from build123d import *

# Parameters (mm, degrees)
SKETCH1_W           = 14.5
SKETCH1_H           = 14.5
BOSS_EXTRUDE1_DEPTH = 24.6
CUT_EXTRUDE1_DEPTH  = 10
SKETCH4_R           = 4
BOSS_EXTRUDE2_DEPTH = 2
FILLET1_R           = 0.5
SKETCH6_W           = 8.45
SKETCH6_H           = 14.5
BOSS_EXTRUDE3_DEPTH = 5
SKETCH7_W           = 6
SKETCH7_H           = 2
CUT_EXTRUDE2_DEPTH  = 5
SKETCH8_R           = 0.55
CUT_EXTRUDE3_DEPTH  = 33.586807146
SKETCH9_R           = 1
CUT_EXTRUDE4_DEPTH  = 29.855891946


with BuildPart() as part:
    # Sketch1 → Boss-Extrude1 (new body)
    with BuildSketch(Plane(origin=(0, 0, 0), x_dir=(1, 0, 0), z_dir=(0, 1, 0))):
        Rectangle(SKETCH1_W, SKETCH1_H)
    extrude(amount=BOSS_EXTRUDE1_DEPTH)

    # Sketch2 → Cut-Extrude1 (cut, symmetric)
    with BuildSketch(Plane(origin=(0, 0, 0), x_dir=(0, 0, -1), z_dir=(1, 0, 0))):
        Polygon((-2, 24.6), (2, 24.6), (4.020725942, 21.1), (-4.020725942, 21.1), align=None)
    extrude(amount=CUT_EXTRUDE1_DEPTH, both=True, mode=Mode.SUBTRACT)

    # Sketch4 → Boss-Extrude2 (add)
    with BuildSketch(Plane.XZ):
        with Locations(Location((0, 0, 0), (0, 0, 270))):
            Circle(SKETCH4_R)
    extrude(amount=BOSS_EXTRUDE2_DEPTH)

    # Sketch3 → Cut-Revolve1 (revolve, cut)
    with BuildSketch(Plane(origin=(0, 0, 0), x_dir=(0, 0, -1), z_dir=(1, 0, 0))):
        with BuildLine():
            Line((3.302, 0), (3.302, -3.302))
            Line((3.302, -3.302), (0, -3.302))
            Line((0, -3.302), (0, 0))
            Line((0, 0), (0, 3.302))
            ThreePointArc((0, 3.302), (2.334866591, 2.334866591), (3.302, 0))
        make_face()
    revolve(axis=Axis((0, 0, 0), (0, 1, 0)), mode=Mode.SUBTRACT)

    # Fillet1
    fillet1_edges = [part.edges().sort_by_distance(p)[0] for p in [
        (0, 24.6, 2),
        (0, 24.6, -2),
        (0, 21.1, -4.020725942),
        (0, 21.1, 4.020725942),
    ]]
    fillet(fillet1_edges, radius=FILLET1_R)

    # Sketch6 → Boss-Extrude3 (add)
    with BuildSketch(Plane(origin=(0, 0, 0), x_dir=(1, 0, 0), z_dir=(0, 1, 0))):
        with Locations((11.475, 0)):
            Rectangle(SKETCH6_W, SKETCH6_H)
        with Locations((-11.475, 0)):
            Rectangle(SKETCH6_W, SKETCH6_H)
    extrude(amount=BOSS_EXTRUDE3_DEPTH)

    # Sketch7 → Cut-Extrude2 (cut)
    with BuildSketch(Plane.XZ):
        with Locations((10.7, 4.125)):
            Rectangle(SKETCH7_W, SKETCH7_H)
        with Locations((-10.7, -4.125)):
            Rectangle(SKETCH7_W, SKETCH7_H)
    extrude(amount=-CUT_EXTRUDE2_DEPTH, mode=Mode.SUBTRACT)

    # Sketch8 → Cut-Extrude3 (cut, through all)
    with BuildSketch(Plane(origin=(0, 0, -7.25), x_dir=(-1, 0, 0), z_dir=(0, 0, -1))):
        with Locations((-10.7, 2.5)):
            Circle(SKETCH8_R)
        with Locations((10.7, 2.5)):
            Circle(SKETCH8_R)
    extrude(amount=-CUT_EXTRUDE3_DEPTH, mode=Mode.SUBTRACT)

    # Sketch9 → Cut-Extrude4 (cut, through all)
    with BuildSketch(Plane(origin=(0, 21.1, 0), x_dir=(1, 0, 0), z_dir=(0, 1, 0))):
        with Locations(Location((0, 0, 0), (0, 0, 270))):
            Circle(SKETCH9_R)
    extrude(amount=-CUT_EXTRUDE4_DEPTH, mode=Mode.SUBTRACT)


solid = part.part
For this review, take the finished solid that the model builds, in its own axes (mm). A direction names the side the tool comes from. Give positions to 0.01 mm unless a question says otherwise; leave off trailing zeros. Loops run counter-clockwise (first coordinate to the right, second up) from the corner with the lowest first, then second, coordinate; pieces in that order, holes last. Notation, with made-up numbers: M 10.25,-1.5 L 63.25,-1.5 A22 cw 63.25,18.5 Z; hole C 86,36.25 d10. An arc over 180 degrees is marked long. Answer as a JSON object with one key per item and string values. Group by question number.
Q1. Tool access review of faces 5 (the flat face through (-7.7, 2, -4)), 6 (the flat face through (-7.25, 15, 0)), 7 (the flat face through (7.25, 15, 0)), 8 (the flat face through (0.101, 22.836, 3.018)), 9 (the cylindrical face through (-3.905, -0.986, 0.867)): name each direction out of +Z, -Z, +X, -X, +Y, -Y from which nothing blocks a thin tool from reaching the whole face with its end or side.
Q2. Add section A-A on z = 0. Give the boundary of the cut face in (x, y).
Q3. Add section B-B on x = 10.7. Give the boundary of the cut face in (y, z) (3 decimals), and give its area (4 significant figures).
Q4. Add section C-C on z = 4.5. Give the boundary of the cut face in (x, y).
Q5. Mouldability with a two-part tool opening along Y and no side actions: class faces 1 (the flat face through (-12, 5, 2)), 2 (the flat face through (0.101, 22.864, -3.002)), 3 (the flat face through (0.1, 21.1, 1.4)), 4 (the flat face through (0, 9, 7.25)) as +Y half, -Y half, draft (parallel to the pull), parting line (faces both ways), or undercut.
Q6. Insertion check: P1, Ø1.8, axis at x = -10.7, y = 2.5, coming from the +Z side; P2, Ø1, axis at x = 3.5, z = 3, coming from the -Y side; P3, Ø7, axis at y = 19, z = 3.5, coming from the -X side; P4, Ø2, axis at y = 19.5, z = -0.5, coming from the +X side. Each pin has a flat end and moves straight along its axis. Give the tip position at first contact, or say it passes through.
Q7. Add section D-D on x = -12. Give the boundary of the cut face in (y, z) (3 decimals), and give its area (3 significant figures).
Q8. For probe 1 along Z at (x, y) = (-10, 3.5) (3 decimals); probe 2 along Z at (x, y) = (10.5, 3.25) (3 decimals); probe 3 along Y at (x, z) = (-13.5, -5.75), list the stretches that pass through material, from the lowest coordinate up. Write a range as [from, to].
Checked values:
{
 "1": {"face 5": "+Y, -Y", "face 6": "+Z, -Z, -X, +Y", "face 7": "+Z, -Z, +X, +Y", "face 8": "+X, -X", "face 9": "-Y"},
 "2": {"outline": "M -15.7,0 L -4,0 L -4,-2 L -3.3,-2 L -3.3,0 A3.3 cw -1,3.15 L -1,21.1 L -7.25,21.1 L -7.25,5 L -15.7,5 Z; M 1,3.15 A3.3 cw 3.3,0 L 3.3,-2 L 4,-2 L 4,0 L 15.7,0 L 15.7,5 L 7.25,5 L 7.25,21.1 L 1,21.1 Z; hole C -10.7,2.5 d1.1; hole C 10.7,2.5 d1.1"},
 "3": {"outline": "M 0,-7.25 L 1.95,-7.25 L 1.95,3.125 L 0,3.125 Z; M 0,5.125 L 1.95,5.125 L 1.95,7.25 L 0,7.25 Z; M 3.05,-7.25 L 5,-7.25 L 5,3.125 L 3.05,3.125 Z; M 3.05,5.125 L 5,5.125 L 5,7.25 L 3.05,7.25 Z", "area": "48.75 mm²"},
 "4": {"outline": "M -15.7,0 L 7.7,0 L 7.7,5 L 7.25,5 L 7.25,24.6 L -7.25,24.6 L -7.25,5 L -15.7,5 Z; M 13.7,0 L 15.7,0 L 15.7,5 L 13.7,5 Z; hole C -10.7,2.5 d1.1"},
 "5": {"face 1": "+Y half", "face 2": "undercut", "face 3": "undercut", "face 4": "draft"},
 "6": {"P1": "z = 7.25", "P2": "y = 0", "P3": "x = -7.25", "P4": "x = 7.25"},
 "7": {"outline": "M 0,-7.25 L 5,-7.25 L 5,-5.125 L 0,-5.125 Z; M 0,-3.125 L 5,-3.125 L 5,7.25 L 0,7.25 Z", "area": "62.5 mm²"},
 "8": {"probe 1": "[-7.25, -5.125], [-3.125, 7.25]", "probe 2": "[-7.25, 3.125], [5.125, 7.25]", "probe 3": "[0, 5]"}
}
